Part model, mm, in its own coordinate system. A direction names the side the tool comes from. Round coordinates to 2 decimals unless told otherwise and drop trailing zeros. Write each loop counter-clockwise with the first axis right and the second up, starting at its lowest first coordinate (ties: lowest second). Pieces come first, ordered by that corner, then holes.
1) Flat gauge pins, fed straight in: pin 1 (1.5 mm diameter, centred on x = -11, z = -13.5, fed in from -Y); pin 2 (1 mm diameter, centred on y = 7, z = -11.5, fed in from +X); pin 3 (1 mm diameter, centred on y = 12.5, z = 1, fed in from -X); pin 4 (5 mm diameter, centred on y = 9.5, z = 16, fed in from -X). Where does each tip first touch, or does it go through?
2) Saw through at B-B on y = 4.25. Count the separate pieces of the cut face and the enclosed holes in it, and give its area (3 significant figures).
3) Drill centre lines: L1, parallel to X at y = 15.75, z = 0; L2, parallel to Y at x = -9.5, z = -9; L3, parallel to Z at x = -6.5, y = 6.75. Where is each one in solid material? Low to high.
4) Pull direction Z, two halves, no side cores. Call faces 4 (the flat face through (-4, 6, 0)), 5 (the cylindrical face through (-6.007, 13.112, -19.076)), 6 (the flat face through (-16, 5, -9)): +Z half, -Z half, draft (parallel to the pull), parting line (faces both ways), or undercut.
5) Saw through at D-D on y = 18. Write the cut outline in (x, z).
6) Saw through at C-C on z = 1. Write the cut outline in (x, y).
7) Saw through at A-A on x = 0. Write the cut outline in (y, z) (1 decimal).
8) Which spindle directions (+Z, -Z, +X, -X, +Y, -Y) get a long thin tool onto all of the face, cutting with end or side? Do faces 1 (the flat face through (16, 5, 9)), 2 (the flat face through (-16, 5, 9)), 3 (the flat face through (16, 5, -9)). Say none if no direction does.
```python
from build123d import *

# Parameters (mm, degrees)
SCHIZZO2_R               = 3.175
SCHIZZO2_R_2             = 0.5
TAGLIO_ESTRUSIONE1_DEPTH = 10
TAGLIO_ESTRUSIONE2_START = -5
TAGLIO_ESTRUSIONE2_DEPTH = 5


with BuildPart() as part:
    # Schizzo1 → Rivoluzione1 (revolve)
    with BuildSketch(Plane.XY, mode=Mode.PRIVATE) as rivoluzione1_sk:
        Polygon((0, 0), (-20, 0), (-20, 21), (-15.5465, 21), (-15.5465, 6), (0, 6), align=None)
    revolve(rivoluzione1_sk.sketch.rotate(Axis((0, 0, 0), (0, 1, 0)), 270), axis=Axis((0, 0, 0), (0, 1, 0)))

    # Schizzo2 → Taglio-Estrusione1 (cut)
    with BuildSketch(Plane.XZ):
        with Locations(Location((0, 0, 0), (0, 0, 270))):
            Circle(SCHIZZO2_R)
        with Locations(Location((10, 0, 0), (0, 0, 270))):
            Circle(SCHIZZO2_R_2)
    extrude(amount=-TAGLIO_ESTRUSIONE1_DEPTH, mode=Mode.SUBTRACT)

    # Schizzo5 → Taglio-Estrusione2 (cut)
    with BuildSketch(Plane(origin=(0, 0, 0), x_dir=(-1, 0, 0), z_dir=(0, -1, 0)).offset(TAGLIO_ESTRUSIONE2_START)):
        with BuildLine():
            Line((-10, 17.320508076), (10, 17.320508076))
            ThreePointArc((10, 17.320508076), (0, 20), (-10, 17.320508076))
        make_face()
        with BuildLine():
            ThreePointArc((20, 0), (17.320508076, 10), (10, 17.320508076))
            Line((10, 17.320508076), (20, 0))
        make_face()
        with BuildLine():
            ThreePointArc((10, -17.320508076), (17.320508076, -10), (20, 0))
            Line((20, 0), (10, -17.320508076))
        make_face()
        with BuildLine():
            ThreePointArc((-10, -17.320508076), (0, -20), (10, -17.320508076))
            Line((10, -17.320508076), (-10, -17.320508076))
        make_face()
        with BuildLine():
            Line((-10, -17.320508076), (-20, 0))
            ThreePointArc((-20, 0), (-17.320508076, -10), (-10, -17.320508076))
        make_face()
        with BuildLine():
            Line((-20, 0), (-10, 17.320508076))
            ThreePointArc((-10, 17.320508076), (-17.320508076, 10), (-20, 0))
        make_face()
    extrude(amount=TAGLIO_ESTRUSIONE2_DEPTH, mode=Mode.SUBTRACT)


solid = part.part
```
Completed:
1. pin 1: stops at y = 0
1. pin 2: stops at x = 16.7
1. pin 3: stops at x = -19.99
1. pin 4: stops at x = -14.76
2. separate pieces: 1
2. enclosed holes: 2
2. area: 1,010 mm2
3. L1: x = -20 to -15.55, 15.55 to 20
3. L2: y = 0 to 6
3. L3: z = -18.91 to -14.12, 14.12 to 18.91
4. face 4: undercut
4. face 5: parting line
4. face 6: draft
5. outline: circle Ø40 at (0, 0); hole circle Ø31.09 at (0, 0)
6. outline: (-19.97, 5) - (-19.42, 5) - (-19.42, 0) - (-3.01, 0) - (-3.01, 6) - (-15.51, 6) - (-15.51, 21) - (-19.97, 21) - close; (3.01, 0) - (19.42, 0) - (19.42, 5) - (19.97, 5) - (19.97, 21) - (15.51, 21) - (15.51, 6) - (3.01, 6) - close
7. outline: (0, -17.3) - (5, -17.3) - (5, -20) - (21, -20) - (21, -15.5) - (6, -15.5) - (6, -3.2) - (0, -3.2) - close; (0, 3.2) - (6, 3.2) - (6, 15.5) - (21, 15.5) - (21, 20) - (5, 20) - (5, 17.3) - (0, 17.3) - close
8. face 1: +Z, +X, -Y
8. face 2: +Z, -X, -Y
8. face 3: -Z, +X, -Y
